```python
from build123d import *

# Parameters (mm, degrees)
SKETCH1_R           = 4.7625
BOSS_EXTRUDE1_DEPTH = 3.175


with BuildPart() as part:
    # Sketch1 → Boss-Extrude1 (new, symmetric)
    with BuildSketch(Plane.XY):
        with BuildLine():
            Line((-602.329569775, -14.917620355), (0, -234.147654972))
            Line((0, -234.147654972), (602.329569775, -14.917620355))
            ThreePointArc((602.329569775, -14.917620355), (611.817620355, 5.429569775), (591.470430225, 14.917620355))
            Line((591.470430225, 14.917620355), (0, -200.360010695))
            Line((0, -200.360010695), (-591.470430225, 14.917620355))
            ThreePointArc((-591.470430225, 14.917620355), (-611.817620355, 5.429569775), (-602.329569775, -14.917620355))
        make_face()
        with Locations((-596.9, 0)):
            Circle(SKETCH1_R, mode=Mode.SUBTRACT)
        with Locations((596.9, 0)):
            Circle(SKETCH1_R, mode=Mode.SUBTRACT)
        with Locations((-167.272533777, -156.371609528)):
            Circle(SKETCH1_R, mode=Mode.SUBTRACT)
    extrude(amount=BOSS_EXTRUDE1_DEPTH, both=True)


solid = part.part
```
Model file for the job. Use its own axes, mm. A direction names the side the tool comes from. Coordinates: 2 decimals unless noted, no trailing zeros. Loops run counter-clockwise (first coordinate to the right, second up) from the corner with the lowest first, then second, coordinate; pieces in that order, holes last. Notation, with made-up numbers: M 45,35.25 L 56,35.25 A17 ccw 56,40.25 Z; hole C 87.25,81 d7. An arc over 180 degrees is marked long. Use CSV: the item, a comma, the result in double quotes. Start each with the question number.
1. Tool access for faces 1 (the flat face through (-3, -201, 3.175)), 2 (the flat face through (299.876, -91.214, 0.044)): list every direction of +Z, -Z, +X, -X, +Y, -Y with a clear straight run to the whole face (end or side of a thin tool).
2. Two-plate mould, pull along X, no slides. Class faces 3 (the flat face through (-305.38, -123, 0.04)), 4 (the flat face through (-3, -201, -3.175)), 5 (the flat face through (296.948, -126.067, 0.044)), 6 (the flat face through (-291.59, -94.23, 0.04)): pulls with the +X half, pulls with the -X half, needs draft (parallel to the pull), parting line crosses it, or undercut.
3. Band-saw the part on B-B, the plane z = 1.5. Give the number of separate pieces and of enclosed holes in the cut face, then the cut area to 3 significant figures.
4. Band-saw the part on C-C, the plane x = 307. List the corners of the cut face in (y, z) (3 decimals), then the cut area to 3 significant figures.
5. Probe probe 1 along Y at (x, z) = (-596.9, 1) (1 decimal); probe 2 along Y at (x, z) = (495.5, 0.25); probe 3 along Y at (x, z) = (-510.5, 1). List the from-to ranges inside material, lowest first. Write a range as [from, to].
6. Band-saw the part on A-A, the plane y = -106. List the corners of the cut face in (x, z) (3 decimals).
7. Flat gauge pins, fed straight in: pin 1 (2 mm diameter, centred on x = -359.5, z = 0.5, fed in from +Y); pin 2 (15 mm diameter, centred on x = 596.9, y = 0, fed in from -Z) (3 decimals). Where does each tip first touch, or does it go through?
Entries:
1,face 1,"+Z, +X, -X, +Y, -Y"
1,face 2,"+Z, -Z, +Y"
2,face 3,"pulls with the -X half"
2,face 4,"needs draft"
2,face 5,"pulls with the +X half"
2,face 6,"undercut"
3,separate pieces,"1"
3,enclosed holes,"3"
3,area,"40,900 mm2"
4,outline,"M -122.409,-3.175 L -88.621,-3.175 L -88.621,3.175 L -122.409,3.175 Z"
4,area,"215 mm2"
5,probe 1,"y = [-16.9, -4.8], [4.8, 15.9]"
5,probe 2,"y = [-53.8, -20.01]"
5,probe 3,"y = [-48.34, -14.55]"
6,outline,"M -352.083,-3.175 L -259.252,-3.175 L -259.252,3.175 L -352.083,3.175 Z; M 259.252,-3.175 L 352.083,-3.175 L 352.083,3.175 L 259.252,3.175 Z"
7,pin 1,"stops at y = -69.15"
7,pin 2,"stops at z = -3.175"
